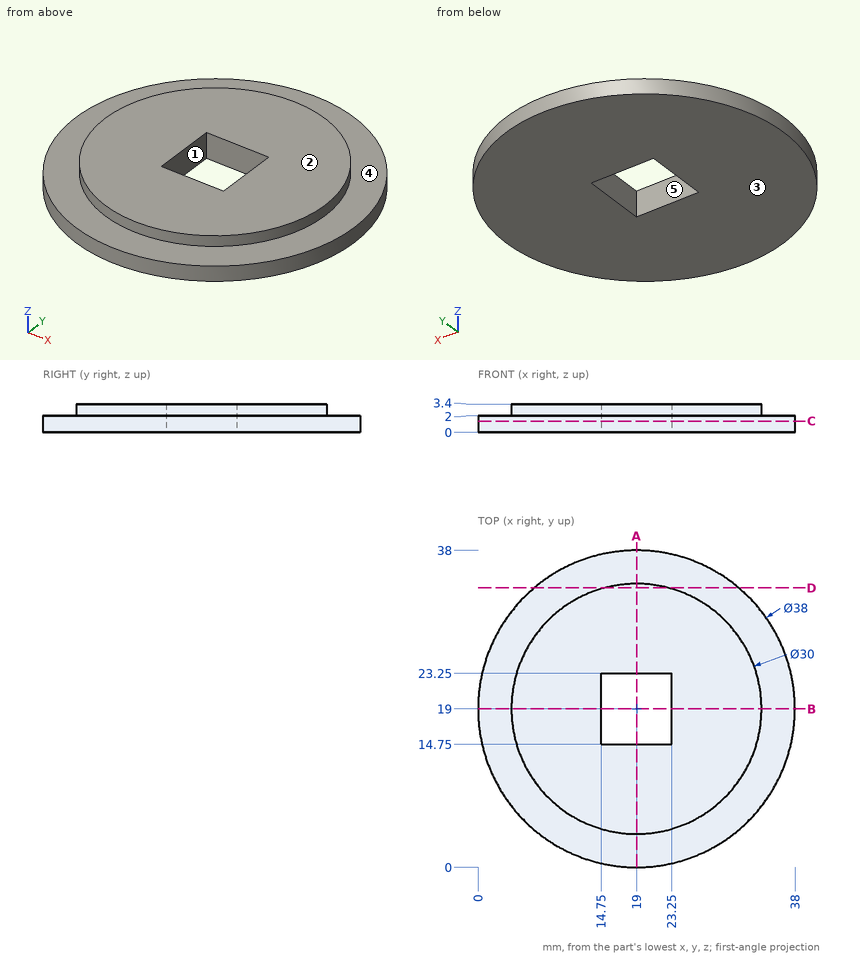
Geometry: see drawing. Coordinates: mm, zero at the bounding-box minimum. A direction names the side the tool comes from. Coordinates: 2 decimals unless noted, no trailing zeros. Loops run counter-clockwise (first coordinate to the right, second up) from the corner with the lowest first, then second, coordinate; pieces in that order, holes last. Notation, with made-up numbers: (-32.75, 86.5) - (-28.75, 86.5) arc R29 ccw to (-28.75, 107.5) - close; hole circle Ø11 at (17, 1). An arc over 180 degrees is marked (long way). Put each result on its own line as item: value. Start each with the question number.
Q1. Pull-direction query (X, two-part tool) for the marked faces 1 and 2; classes: released by +X, released by -X, zero draft, split by the parting line, or undercut.
Q2. Cut plane D-D, the plane y = 33.5. Return loops of the section in (x, z).
Q3. Pin query (flat end, axial travel): pin 1 Ø1 at (x, z) = (20, 2) entering from -Y; pin 2 Ø2 at (y, z) = (16, 2) entering from -X; pin 3 Ø2 at (x, z) = (9, 2.5) entering from +Y. Return the tip coordinate at first contact, or that it passes through.
Q4. Set-up query: the marked faces 3, 4 and 5. Return all of +Z, -Z, +X, -X, +Y, -Y with unobstructed straight access to the full face (end or side cutting, diameter ignored); none if empty.
Q5. Cut plane A-A, the plane x = 19. Return loops of the section in (y, z), and give its area (3 significant figures).
Q6. Cut plane C-C, the plane z = 1.35. Return loops of the section in (x, y).
Q7. Line query: line 1 (Y direction, x = 19.5, z = 3.05); line 2 (Y direction, x = 18.5, z = 1.2); line 3 (X direction, y = 15.5, z = 1.1). Output: solid intervals per line, ascending.
Filled sheet:
1. face 1: undercut
1. face 2: zero draft
2. outline: (6.72, 0) - (31.28, 0) - (31.28, 2) - (22.84, 2) - (22.84, 3.4) - (15.16, 3.4) - (15.16, 2) - (6.72, 2) - close
3. pin 1: y = 0.01
3. pin 2: x = 0.11
3. pin 3: y = 35.66
4. face 3: -Z, +X, -X, +Y, -Y
4. face 4: +Z
4. face 5: +Z, -Z
5. outline: (0, 0) - (14.75, 0) - (14.75, 3.4) - (4, 3.4) - (4, 2) - (0, 2) - close; (23.25, 0) - (38, 0) - (38, 2) - (34, 2) - (34, 3.4) - (23.25, 3.4) - close
5. area: 89.1 mm²
6. outline: circle Ø38 at (19, 19); hole (14.75, 14.75) - (23.25, 14.75) - (23.25, 23.25) - (14.75, 23.25) - close
7. line 1: 4.01 to 14.75, 23.25 to 33.99
7. line 2: 0.01 to 14.75, 23.25 to 37.99
7. line 3: 0.33 to 14.75, 23.25 to 37.67
